```python
from build123d import *

# Parameters (mm, degrees)
SKETCH_1_W      = 65
SKETCH_1_H      = 56
SKETCH_1_R      = 1.25
EXTRUDE_1_DEPTH = 13.8
SKETCH_2_W      = 5
SKETCH_2_H      = 5.72
EXTRUDE_2_DEPTH = 13.8


with BuildPart() as part:
    # 草图1 → 凸台-拉伸1 (new body)
    with BuildSketch(Plane(origin=(0, 0, 0), x_dir=(1, 0, 0), z_dir=(0, 1, 0))):
        Rectangle(SKETCH_1_W, SKETCH_1_H)
        with Locations(Location((-29, 24.5, 0), (0, 0, 90))):
            Circle(SKETCH_1_R, mode=Mode.SUBTRACT)
        with Locations(Location((29, 24.5, 0), (0, 0, 90))):
            Circle(SKETCH_1_R, mode=Mode.SUBTRACT)
        with Locations(Location((29, -24.5, 0), (0, 0, 90))):
            Circle(SKETCH_1_R, mode=Mode.SUBTRACT)
        with Locations(Location((-29, -24.5, 0), (0, 0, 90))):
            Circle(SKETCH_1_R, mode=Mode.SUBTRACT)
    extrude(amount=EXTRUDE_1_DEPTH)

    # 草图2 → 凸台-拉伸2 (add)
    with BuildSketch(Plane(origin=(0, 13.8, 0), x_dir=(1, 0, 0), z_dir=(0, 1, 0))):
        with Locations((18, 30.86)):
            Rectangle(SKETCH_2_W, SKETCH_2_H)
    extrude(amount=-EXTRUDE_2_DEPTH)


solid = part.part
```
The listing builds one solid part. Answer for the finished solid, in the listing's coordinates (mm). A direction names the side the tool comes from. Give positions to 0.01 mm unless a question says otherwise; leave off trailing zeros. Order: outer loops, then holes, each group sorted by start corner. A loop starts at its lowest first (then second) coordinate and runs counter-clockwise, first axis right, second up. Notation, with made-up numbers: (57.25, 22) - (99.25, 22) arc R27 cw to (99.25, 43) - close; hole circle Ø2 at (9.25, 22). An arc over 180 degrees is marked (long way). Answer in a Markdown table with one row per item. Add a question column.
Q1. The part is cut by section A-A (x = 29). Determine the outline of the cut face in (y, z), then the cut area to 3 significant figures.
Q2. Find the intervals of material crossed by line 1 along Z through (x, y) = (29, 6); line 2 along X through (y, z) = (8, -24.5); line 3 along Z through (x, y) = (-9, 11.75), in increasing order. Write a range as [from, to].
Q3. Which of the six approach directions +Z, -Z, +X, -X, +Y, -Y give full straight-line access (tool end or side, diameter ignored) to faces 1 (the cylindrical face through (-28.521, 6.803, -25.655)), 2 (the flat face through (26, 7, -28)), 3 (the flat face through (-9, 7, -28))?
Q4. Given P1, Ø2, axis at x = -29, z = 24.5, coming from the -Y side; P2, Ø4, axis at x = -11, y = 7.5, coming from the -Z side, each flat-ended and moving along its own axis, determine where each tip first touches the part or whether it passes through.
Q5. The part is cut by section B-B (z = -24.5). Determine the outline of the cut face in (x, y), then the cut area to 3 significant figures.
Q6. For a pull along Z with two mould halves and no side action, classify faces 4 (the cylindrical face through (-28.521, 6.803, 23.345)), 5 (the flat face through (20.5, 7, -31)), 6 (the flat face through (0, 7, 28)), 7 (the cylindrical face through (27.946, 6.803, -25.172)) as released by +Z, released by -Z, zero draft, split by the parting line, or undercut.
Q7. The part is cut by section C-C (y = 7.75). Determine the outline of the cut face in (x, z), then the cut area to 3 significant figures.
Determined:
| question | item | result |
|---|---|---|
| 1 | outline | (0, -28) - (13.8, -28) - (13.8, -25.75) - (0, -25.75) - close; (0, -23.25) - (13.8, -23.25) - (13.8, 23.25) - (0, 23.25) - close; (0, 25.75) - (13.8, 25.75) - (13.8, 28) - (0, 28) - close |
| 1 | area | 704 mm² |
| 2 | line 1 | z = [-28, -25.75], [-23.25, 23.25], [25.75, 28] |
| 2 | line 2 | x = [-32.5, -30.25], [-27.75, 27.75], [30.25, 32.5] |
| 2 | line 3 | z = [-28, 28] |
| 3 | face 1 | +Y, -Y |
| 3 | face 2 | -Z, +X, +Y, -Y |
| 3 | face 3 | -Z, -X, +Y, -Y |
| 4 | P1 | passes through |
| 4 | P2 | stops at z = -28 |
| 5 | outline | (-32.5, 0) - (-30.25, 0) - (-30.25, 13.8) - (-32.5, 13.8) - close; (-27.75, 0) - (27.75, 0) - (27.75, 13.8) - (-27.75, 13.8) - close; (30.25, 0) - (32.5, 0) - (32.5, 13.8) - (30.25, 13.8) - close |
| 5 | area | 828 mm² |
| 6 | face 4 | undercut |
| 6 | face 5 | zero draft |
| 6 | face 6 | released by +Z |
| 6 | face 7 | undercut |
| 7 | outline | (-32.5, -28) - (15.5, -28) - (15.5, -33.72) - (20.5, -33.72) - (20.5, -28) - (32.5, -28) - (32.5, 28) - (-32.5, 28) - close; hole circle Ø2.5 at (-29, -24.5); hole circle Ø2.5 at (-29, 24.5); hole circle Ø2.5 at (29, -24.5); hole circle Ø2.5 at (29, 24.5) |
| 7 | area | 3,650 mm² |
